Input: part model. Units: mm. Frame: model coordinates. A direction names the side the tool comes from. Coordinates: 2 decimals unless noted, no trailing zeros. Order: outer loops, then holes, each group sorted by start corner. A loop starts at its lowest first (then second) coordinate and runs counter-clockwise, first axis right, second up. Notation, with made-up numbers: (13, 35) -> (72, 35) arc R28 ccw to (72, 73) -> close; hole circle Ø2 at (86, -28). An arc over 180 degrees is marked (long way). Use one line per item in the form item = value. Start each with the question number.
1) Section query B-B on z = 1.1. Output: boundary loops of the cut face in (x, y).
2) Section query C-C on x = 33.5. Output: boundary loops of the cut face in (y, z).
3) Access query for faces 1 (the cylindrical face through (1.669, -32.974, 1.232)), 2 (the flat face through (29, -9, 0)). Directions: +Z, -Z, +X, -X, +Y, -Y. A direction counts if a zero-diameter tool reaches every point of the face in a straight line with its end or side. Return the directions, or none.
4) Ray query, line 1 along Y through (x, z) = (0, 0.6); line 2 along Z through (x, y) = (-3, -10); line 3 along X through (y, z) = (1, -0.55). Return the intervals inside material, ascending.
5) Pin query (flat end, axial travel): pin 1 (3 mm diameter, centred on x = 0, y = -33.5, fed in from -Z); pin 2 (6 mm diameter, centred on x = 0, y = 0, fed in from +Z); pin 3 (7.5 mm diameter, centred on x = -5.5, y = 6, fed in from -Z); pin 4 (1.5 mm diameter, centred on x = -9.5, z = 1.5, fed in from +Y). Return the tip coordinate at first contact, or that it passes through.
6) Section query A-A on x = 0. Output: boundary loops of the cut face in (y, z).
7) Draft query along X for faces 3 (the cylindrical face through (0.81, 31.95, 1.23)), 4 (the flat face through (-1, -9, 2.5)), 5 (the cylindrical face through (-27.574, -11.433, -0.493)). Return one class per face: pulls with the +X half, pulls with the -X half, needs draft (parallel to the pull), parting line crosses it, or undercut.
from build123d import *

# Parameters (mm, degrees)
SKETCH1_R           = 45
SKETCH1_R_2         = 2.25
SKETCH1_R_3         = 1.75
BOSS_EXTRUDE1_DEPTH = 2.5
SKETCH2_R           = 29.85
SKETCH2_R_2         = 12.65
BOSS_EXTRUDE2_DEPTH = 1


with BuildPart() as part:
    # Sketch1 → Boss-Extrude1 (new body)
    with BuildSketch(Plane.XY):
        Circle(SKETCH1_R)
        Circle(SKETCH1_R_2, mode=Mode.SUBTRACT)
        with Locations((0, 33.5)):
            Circle(SKETCH1_R_3, mode=Mode.SUBTRACT)
        with Locations((33.5, 0)):
            Circle(SKETCH1_R_3, mode=Mode.SUBTRACT)
        with Locations((0, -33.5)):
            Circle(SKETCH1_R_3, mode=Mode.SUBTRACT)
        with Locations((-33.5, 0)):
            Circle(SKETCH1_R_3, mode=Mode.SUBTRACT)
    extrude(amount=BOSS_EXTRUDE1_DEPTH)

    # Sketch2 → Boss-Extrude2 (add)
    with BuildSketch(Plane(origin=(0, 0, 0), x_dir=(-1, 0, 0), z_dir=(0, 0, -1))):
        Circle(SKETCH2_R)
        Circle(SKETCH2_R_2, mode=Mode.SUBTRACT)
    extrude(amount=BOSS_EXTRUDE2_DEPTH)


solid = part.part
Answers below:
q1.outline = circle Ø90 at (0, 0); hole circle Ø3.5 at (-33.5, 0); hole circle Ø4.5 at (0, 0); hole circle Ø3.5 at (0, -33.5); hole circle Ø3.5 at (0, 33.5); hole circle Ø3.5 at (33.5, 0)
q2.outline = (-30.05, 0) -> (-1.75, 0) -> (-1.75, 2.5) -> (-30.05, 2.5) -> close; (1.75, 0) -> (30.05, 0) -> (30.05, 2.5) -> (1.75, 2.5) -> close
q3.face_1 = +Z, -Z
q3.face_2 = -Z
q4.line_1 = -45 to -35.25, -31.75 to -2.25, 2.25 to 31.75, 35.25 to 45
q4.line_2 = 0 to 2.5
q4.line_3 = -29.83 to -12.61, 12.61 to 29.83
q5.pin_1 = through
q5.pin_2 = 2.5
q5.pin_3 = 0
q5.pin_4 = 44.14
q6.outline = (-45, 0) -> (-35.25, 0) -> (-35.25, 2.5) -> (-45, 2.5) -> close; (-31.75, 0) -> (-29.85, 0) -> (-29.85, -1) -> (-12.65, -1) -> (-12.65, 0) -> (-2.25, 0) -> (-2.25, 2.5) -> (-31.75, 2.5) -> close; (2.25, 0) -> (12.65, 0) -> (12.65, -1) -> (29.85, -1) -> (29.85, 0) -> (31.75, 0) -> (31.75, 2.5) -> (2.25, 2.5) -> close; (35.25, 0) -> (45, 0) -> (45, 2.5) -> (35.25, 2.5) -> close
q7.face_3 = undercut
q7.face_4 = needs draft
q7.face_5 = parting line crosses it
